Could you check a few things on this model? Use its own coordinates, in mm. A direction names the side the tool comes from. Give positions to 0.01 mm unless a question says otherwise; leave off trailing zeros. Loops run counter-clockwise (first coordinate to the right, second up) from the corner with the lowest first, then second, coordinate; pieces in that order, holes last. Notation, with made-up numbers: (14, 46.25) - (50, 46.25) arc R23 ccw to (50, 80.25) - close; hole circle Ø2 at (53.5, 28.25). An arc over 180 degrees is marked (long way). Write each question's results on one line, items separated by ' | '. Start each with the question number.
(1) Suppose I cut it at A-A (y = 6.56). Please give me the cut outline in (x, z), and give its area (3 significant figures).
(2) Suppose I cut it at D-D (z = -27.5). Please give me the cut outline in (x, y).
(3) If we mould it in two halves opening along Z, with no side actions, what happens to faces 1 (the face through (13, 113, 30)), 2 (the face through (-6, 100, -14)), 3 (the face through (22.1, 21.5, -13))? For each: released by +Z, released by -Z, zero draft, split by the parting line, or undercut.
(4) I need wall thicknesses on line 1 (Z direction, x = 5.5, y = 19.5); line 2 (Z direction, x = 25, y = 6.56); line 3 (Y direction, x = 27.75, z = -15) (3 decimals). Which ranges of each line are inside material? Lowest first, please.
(5) For pin 1 (5.5 mm diameter, centred on y = 6.56, z = -15, fed in from +X); pin 2 (4 mm diameter, centred on y = 15.06, z = -15, fed in from +X); pin 3 (22 mm diameter, centred on y = 7, z = -12.5, fed in from -X); pin 4 (6 mm diameter, centred on x = 19, z = -28, fed in from -Y), each with a flat end and sliding along its axis, tell me the tip position at first contact or that it passes through.
(6) Suppose I cut it at C-C (x = -3.5). Please give me the cut outline in (y, z), and give its area (3 significant figures).
(7) Suppose I cut it at B-B (z = -15). Count the separate pieces of the cut face and the enclosed holes in it, and give its area (3 significant figures).
(8) On a 3-axis mill with a long thin cutter (end or side, diameter ignored), from which of +Z, -Z, +X, -X, +Y, -Y can I reach the whole of each face in a straight line? I mean faces 4 (the face through (21.035, 27.525, -12.472)), 5 (the face through (-4.535, 123.598, -14.37)), 6 (the face through (10, 31.1, -15)), 7 (the face through (18, 0, -27)). Say none if no direction works.
Autodesk Inventor part; units mm, degrees
ref_plane "Work Plane1" through (0, 0, -15) normal (0, 0, 1) x (1, 0, 0)
ref_plane "YZ Plane" through (0, 0, 0) normal (1, 0, 0) x (0, 1, 0)
ref_plane "XZ Plane" through (0, 0, 0) normal (0, 1, 0) x (-1, 0, 0)
sketch "Sketch1" plane through (0, 0, 0) normal (0, 0, 1) x (1, 0, 0)
  line L0 (0, 0) -> (25, 0)
  line L1 (25, 0) -> (25, 40)
  line L2 (25, 40) -> (0, 40)
  line L3 (0, 40) -> (0, 0)
  dimension "d1" = 25
  dimension "d2" = 40
  dimension "d3" = 25
extrude "Extrusion1" add sketch "Sketch1" against normal blind 30
sketch "Sketch2" plane through (25, 0, 0) normal (1, 0, 0) x (0, 0, -1)
  line L0 (0, 0) -> (30, 0)
  circle A0 centre (15, 6.56) radius 2.46
extrude "Extrusion2" cut sketch "Sketch2" against normal blind 30
sketch "Sketch3" plane through (0, 0, 0) normal (-1, 0, 0) x (0, 0, 1)
  line L0 (0, 0) -> (-30, 0)
  line L1 (-25.05, 0) -> (-4.95, 0)
  line L2 (-4.95, 0) -> (-4.95, 33.12)
  line L3 (-4.95, 33.12) -> (-25.05, 33.12)
  line L4 (-25.05, 33.12) -> (-25.05, 0)
  dimension "d11" = 20.1
extrude "Extrusion3" cut sketch "Sketch3" against normal blind 20
sketch "Sketch4" plane through (0, 0, 0) normal (0, -1, 0) x (1, 0, 0)
  line L0 (20, -4.95) -> (20, -25.05)
  line L1 (20, -15) -> (25, -15)
  line L2 (25, 0) -> (25, -30)
  line L3 (20, -8.025) -> (25, -8.025)
  line L4 (25, -8.025) -> (25, -21.975)
  line L5 (25, -21.975) -> (20, -21.975)
  line L6 (20, -21.975) -> (20, -8.025)
  line L7 (20, -8.025) -> (25, -21.975) construction
  line L8 (25, -8.025) -> (20, -21.975) construction
  line L9 (25, -12.54) -> (25, -17.46)
  point P0 (0, 0)
  point P1 (22.5, -15)
  dimension "d14" = 13.95
extrude "Extrusion4" add sketch "Sketch4" along normal blind 15
sketch "Sketch5" plane through (20, 0, 0) normal (-1, 0, 0) x (0, 0, 1)
  circle A0 centre (-15, 6.56) radius 2.46
  circle A1 centre (-15, 6.56) radius 4.7025
  circle A2 centre (-15, 6.56) radius 2.46
  circle A3 centre (-15, 6.56) radius 2.46
  point P0 (0, 0)
  dimension "d17" = 9.405
extrude "Extrusion5" cut sketch "Sketch5" against normal blind 2.1
sketch "Sketch6" plane through (25, 0, 0) normal (1, 0, 0) x (0, 0, -1)
  circle A0 centre (15, 6.56) radius 4.7025
  line L0 (15, 6.56) -> (15, 23.56)
  circle A1 centre (15, 23.56) radius 2.46
  point P0 (0, 0)
  dimension "d20" = 17
  dimension "d21" = 4.92
extrude "Extrusion6" cut sketch "Sketch6" against normal blind 10 contours A1
sketch "Sketch7" plane through (20, 0, 0) normal (-1, 0, 0) x (0, 0, 1)
  circle A0 centre (-15, 23.56) radius 2.46
  circle A1 centre (-15, 23.56) radius 4.7025
  point P0 (0, 0)
  dimension "d24" = 9.405
extrude "Extrusion7" cut sketch "Sketch7" against normal blind 2.1
sketch "Sketch9" plane through (25, 0, 0) normal (1, 0, 0) x (0, 0, -1)
  circle A0 centre (15, 6.56) radius 2.46
  circle A1 centre (15, 6.56) radius 2.46
  circle A2 centre (15, 23.56) radius 2.46
  circle A3 centre (15, 23.56) radius 2.46
  line L0 (30, 40) -> (30, 0)
  line L1 (30, 0) -> (30, 40)
  line L2 (30, 40) -> (0, 40)
  line L3 (0, 40) -> (0, 0)
  line L4 (0, 0) -> (8.025, 0)
  line L5 (21.975, 0) -> (21.975, -15)
  line L6 (21.975, -15) -> (8.025, -15)
  line L7 (8.025, -15) -> (8.025, 0)
  line L8 (0, 0) -> (8.025, 0)
  line L9 (21.975, 0) -> (30, 0)
extrude "Extrusion8" add sketch "Sketch9" along normal blind 5
sketch "Sketch10" plane through (0, 40, 0) normal (0, 1, 0) x (1, 0, 0)
  line L0 (0, 30) -> (30, 30)
  line L1 (30, 0) -> (0, 0)
  line L2 (0, 30) -> (30, 30)
  line L3 (30, 30) -> (30, 0)
  line L4 (30, 0) -> (0, 0)
  line L5 (0, 0) -> (0, 30)
extrude "Extrusion9" add sketch "Sketch10" along normal blind 30
sketch "Sketch12" plane through (30, 0, 0) normal (1, 0, 0) x (0, 0, -1)
  circle A0 centre (15, 6.56) radius 2.46
  line L0 (15, 6.56) -> (15, 15.06)
  circle A1 centre (15, 15.06) radius 2.525
  point P0 (0, 0)
  dimension "d31" = 8.5
  dimension "d33" = 5.05
extrude "Extrusion10" cut sketch "Sketch12" against normal blind 30 contours A1
sketch "Sketch14" plane through (0, 0, 0) normal (0, 0, 1) x (1, 0, 0)
  line L0 (30, 70) -> (0, 70)
  line L1 (0, 70) -> (0, 85)
  line L2 (30, 0) -> (30, 70)
  line L3 (30, 118) -> (30, 70)
  line L4 (30, 105) -> (30, 100)
  line L5 (-12, 133) -> (15, 133)
  line L6 (-7, 130.5) -> (-12, 133)
  line L7 (-7, 130.5) -> (-2, 116.5)
  line L8 (-7, 102.5) -> (-12, 100)
  line L9 (-7, 102.5) -> (-2, 116.5)
  line L10 (30, 118) -> (15, 133)
  line L11 (0, 100) -> (-12, 100)
  line L12 (0, 100) -> (0, 85)
  point P0 (0, 0)
  dimension "d79" = 12
extrude "Extrusion12" add sketch "Sketch14" against normal blind 30
sketch "Sketch15" plane through (0, 0, -25.05) normal (-1, 0, 0) x (0, 0, 1)
  line L0 (0, 33.12) -> (20.1, 33.12)
  line L1 (20.1, 33.12) -> (20.1, 0)
  line L2 (0, 33.12) -> (20.1, 33.12)
  line L3 (20.1, 33.12) -> (20.1, 31.1)
  line L4 (20.1, 31.1) -> (0, 31.1)
  line L5 (0, 31.1) -> (0, 33.12)
  point P0 (25.05, 0)
  dimension "d57" = 2.02
extrude "Extrusion13" add sketch "Sketch15" against normal blind 20
sketch "Sketch22" plane through (0, 0, 0) normal (0, 0, 1) x (1, 0, 0)
  line L0 (0, 100) -> (-12, 100)
  line L1 (0, 100) -> (-12, 100)
  line L2 (-12, 100) -> (-7, 102.5)
  line L3 (-12, 100) -> (-7, 102.5)
  line L4 (-7, 102.5) -> (-2, 116.5)
  line L5 (-7, 102.5) -> (-2, 116.5)
  line L6 (-2, 116.5) -> (-7, 130.5)
  line L7 (-2, 116.5) -> (-7, 130.5)
  line L8 (-7, 130.5) -> (-12, 133)
  line L9 (-7, 130.5) -> (-12, 133)
  line L10 (-12, 133) -> (15, 133)
  line L11 (-12, 133) -> (15, 133)
  line L12 (15, 133) -> (30, 118)
  line L13 (15, 133) -> (30, 118)
  line L14 (30, 118) -> (30, 93)
  line L15 (30, 0) -> (30, 118)
  line L16 (30, 93) -> (0, 93)
  line L17 (0, 100) -> (0, 0)
  line L18 (0, 93) -> (0, 100)
  dimension "d80" = 25
extrude "Extrusion14" add sketch "Sketch22" along normal blind 30
ref_plane "Work Plane1" through (0, 0, -15) normal (0, 0, 1) x (1, 0, 0)
mirror "Mirror1" about plane through (0, 0, -15) normal (0, 0, 1) of "Extrusion14"
properties part number "rec_b_28mm_x_90mm"
Output values:
1) outline: (0, -30) - (30, -30) - (30, -17.46) - (22.1, -17.46) - (22.1, -19.7) - (20, -19.7) - (20, -25.05) - (0, -25.05) - close; (0, -4.95) - (20, -4.95) - (20, -10.3) - (22.1, -10.3) - (22.1, -12.54) - (30, -12.54) - (30, 0) - (0, 0) - close | area: 439 mm2
2) outline: (-12, 100) - (0, 100) - (0, 0) - (30, 0) - (30, 118) - (15, 133) - (-12, 133) - (-7, 130.5) - (-2, 116.5) - (-7, 102.5) - close
3) face 1: released by +Z | face 2: zero draft | face 3: undercut
4) line 1: -30 to -25.05, -4.95 to 0 | line 2: -30 to -17.46, -12.54 to 0 | line 3: -15 to 4.1, 9.02 to 12.535, 17.585 to 21.1, 26.02 to 120.25
5) pin 1: x = 30 | pin 2: through | pin 3: x = 0 | pin 4: y = 0
6) outline: (100, -60) - (112.3, -60) - (112.3, 30) - (100, 30) - close; (120.7, -60) - (133, -60) - (133, 30) - (120.7, 30) - close | area: 2,210 mm2
7) separate pieces: 4 | enclosed holes: 0 | area: 3,410 mm2
8) face 4: -X | face 5: +Z, -Z, -X | face 6: -X, -Y | face 7: -Z, +X, -X, -Y
